```python
from build123d import *

# Parameters (mm, degrees)
SKETCH1_W           = 16
SKETCH1_H           = 4.25
BOSS_EXTRUDE1_DEPTH = 4.25
SKETCH3_W           = 0.5
SKETCH3_H           = 0.5
BOSS_EXTRUDE2_DEPTH = 3
SKETCH4_W           = 0.5
SKETCH4_H           = 0.5
CUT_EXTRUDE1_DEPTH  = 4


with BuildPart() as part:
    # Sketch1 → Boss-Extrude1 (new body)
    with BuildSketch(Plane(origin=(0, 0, 0), x_dir=(1, 0, 0), z_dir=(0, 1, 0))):
        with Locations((8, -2.125)):
            Rectangle(SKETCH1_W, SKETCH1_H)
    extrude(amount=BOSS_EXTRUDE1_DEPTH)

    # Sketch3 → Boss-Extrude2 (add)
    with BuildSketch(Plane.XZ):
        with Locations((3, 1.125)):
            Rectangle(SKETCH3_W, SKETCH3_H)
        with Locations((1, 1.125)):
            Rectangle(SKETCH3_W, SKETCH3_H)
        with Locations((5, 1.125)):
            Rectangle(SKETCH3_W, SKETCH3_H)
        with Locations((7, 1.125)):
            Rectangle(SKETCH3_W, SKETCH3_H)
        with Locations((9, 1.125)):
            Rectangle(SKETCH3_W, SKETCH3_H)
        with Locations((11, 1.125)):
            Rectangle(SKETCH3_W, SKETCH3_H)
        with Locations((13, 1.125)):
            Rectangle(SKETCH3_W, SKETCH3_H)
        with Locations((15, 1.125)):
            Rectangle(SKETCH3_W, SKETCH3_H)
        with Locations((1, 3.125)):
            Rectangle(SKETCH3_W, SKETCH3_H)
        with Locations((3, 3.125)):
            Rectangle(SKETCH3_W, SKETCH3_H)
        with Locations((5, 3.125)):
            Rectangle(SKETCH3_W, SKETCH3_H)
        with Locations((7, 3.125)):
            Rectangle(SKETCH3_W, SKETCH3_H)
        with Locations((9, 3.125)):
            Rectangle(SKETCH3_W, SKETCH3_H)
        with Locations((11, 3.125)):
            Rectangle(SKETCH3_W, SKETCH3_H)
        with Locations((13, 3.125)):
            Rectangle(SKETCH3_W, SKETCH3_H)
        with Locations((15, 3.125)):
            Rectangle(SKETCH3_W, SKETCH3_H)
    extrude(amount=BOSS_EXTRUDE2_DEPTH)

    # Sketch4 → Cut-Extrude1 (cut)
    with BuildSketch(Plane(origin=(0, 4.25, 0), x_dir=(-1, 0, 0), z_dir=(0, 1, 0))):
        with Locations((-15, 1.125)):
            Rectangle(SKETCH4_W, SKETCH4_H)
        with Locations((-13, 1.125)):
            Rectangle(SKETCH4_W, SKETCH4_H)
        with Locations((-11, 1.125)):
            Rectangle(SKETCH4_W, SKETCH4_H)
        with Locations((-9, 1.125)):
            Rectangle(SKETCH4_W, SKETCH4_H)
        with Locations((-7, 1.125)):
            Rectangle(SKETCH4_W, SKETCH4_H)
        with Locations((-5, 1.125)):
            Rectangle(SKETCH4_W, SKETCH4_H)
        with Locations((-3, 1.125)):
            Rectangle(SKETCH4_W, SKETCH4_H)
        with Locations((-1, 1.125)):
            Rectangle(SKETCH4_W, SKETCH4_H)
        with Locations((-15, 3.125)):
            Rectangle(SKETCH4_W, SKETCH4_H)
        with Locations((-13, 3.125)):
            Rectangle(SKETCH4_W, SKETCH4_H)
        with Locations((-11, 3.125)):
            Rectangle(SKETCH4_W, SKETCH4_H)
        with Locations((-9, 3.125)):
            Rectangle(SKETCH4_W, SKETCH4_H)
        with Locations((-7, 3.125)):
            Rectangle(SKETCH4_W, SKETCH4_H)
        with Locations((-5, 3.125)):
            Rectangle(SKETCH4_W, SKETCH4_H)
        with Locations((-3, 3.125)):
            Rectangle(SKETCH4_W, SKETCH4_H)
        with Locations((-1, 3.125)):
            Rectangle(SKETCH4_W, SKETCH4_H)
    extrude(amount=-CUT_EXTRUDE1_DEPTH, mode=Mode.SUBTRACT)


solid = part.part
```
Design review of the part built by this model. Coordinates are the model's own, in mm. Give positions to 0.01 mm unless a question says otherwise; leave off trailing zeros. Loops run counter-clockwise (first coordinate to the right, second up) from the corner with the lowest first, then second, coordinate; pieces in that order, holes last. Notation, with made-up numbers: M 35,52.5 L 68,52.5 A14 cw 68,63.5 Z; hole C 89.5,-4.75 d3. An arc over 180 degrees is marked long. Return JSON: item names as keys, results as strings. Group by question number.
Item 1: We need section A-A (y = -0.5). Give the number of separate pieces and of enclosed holes in the cut face, and give its area (3 significant figures).
Item 2: For probe 1 along Z at (x, y) = (1, 0.5) (3 decimals); probe 2 along Z at (x, y) = (15, -1.5) (3 decimals); probe 3 along Y at (x, z) = (11, 1.65), list the stretches that pass through material, from the lowest coordinate up.
Item 3: We need section B-B (z = 2.5). Give the boundary of the cut face in (x, y).
Item 4: Mouldability with a two-part tool opening along Z and no side actions: class faces 1 (the flat face through (8, 0, 2)), 2 (the flat face through (8, 2, 4.25)), 3 (the flat face through (16, 2, 2)) as released by +Z, released by -Z, zero draft, split by the parting line, or undercut.
Item 5: Insertion check: pin 1 Ø0.6 at (x, y) = (15, -1.5) entering from +Z (3 decimals); pin 2 Ø0.6 at (y, z) = (-1.5, 3) entering from +X. Each pin has a flat end and moves straight along its axis. Give the tip position at first contact, or say it passes through.
Item 6: We need section C-C (x = 2). Give the boundary of the cut face in (y, z).
Output:
{
 "1": {"separate pieces": "16", "enclosed holes": "0", "area": "4.00 mm^2"},
 "2": {"probe 1": "z = 0 to 0.875, 1.375 to 2.875, 3.375 to 4.25", "probe 2": "z = 0.875 to 1.375, 2.875 to 3.375", "probe 3": "y = 0 to 4.25"},
 "3": {"outline": "M 0,0 L 16,0 L 16,4.25 L 0,4.25 Z"},
 "4": {"face 1": "undercut", "face 2": "released by +Z", "face 3": "zero draft"},
 "5": {"pin 1": "stops at z = 3.375", "pin 2": "stops at x = 15.25"},
 "6": {"outline": "M 0,0 L 4.25,0 L 4.25,4.25 L 0,4.25 Z"}
}
